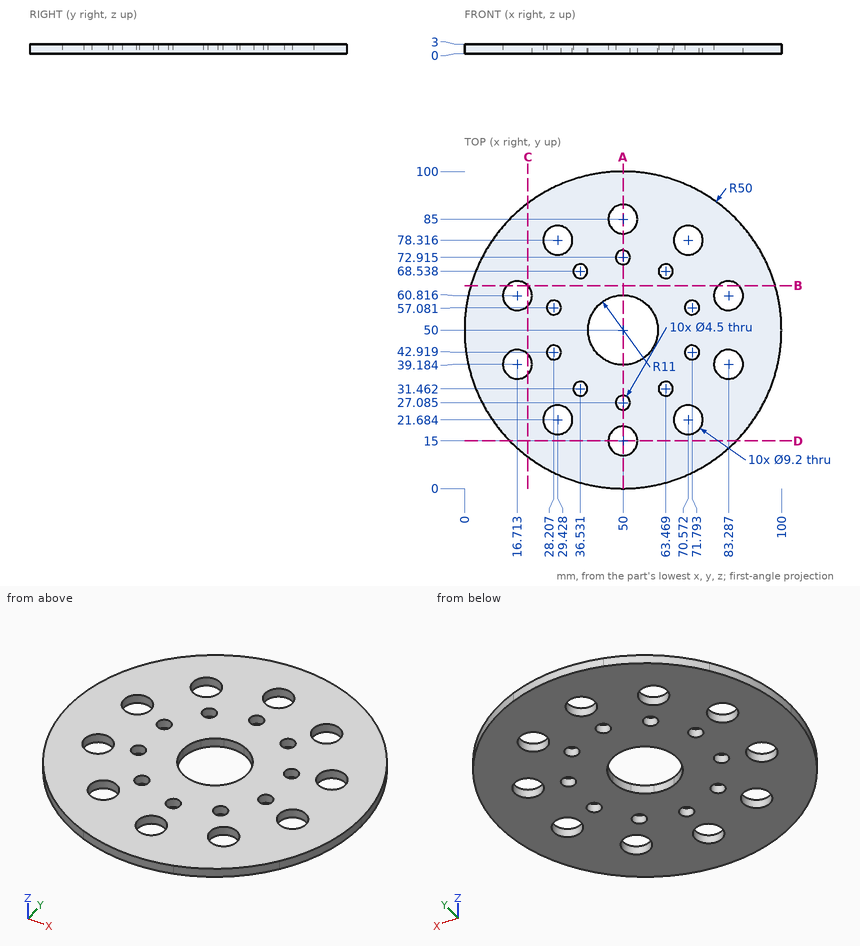
Print and shaded views of the part. All mm, measured from the part's lowest x, y and z. Coordinates: 2 decimals unless noted, no trailing zeros. Loops run counter-clockwise (first coordinate to the right, second up) from the corner with the lowest first, then second, coordinate; pieces in that order, holes last. Notation, with made-up numbers: (59.25, 68) - (88.25, 68) arc R22 cw to (88.25, 102) - close; hole circle Ø2 at (17.25, -38.5). An arc over 180 degrees is marked (long way). Use one line per item in the form item = value. Start each with the question number.
1) Drill centre lines: L1, parallel to Y at x = 50, z = 2.35 (1 decimal); L2, parallel to X at y = 75.5, z = 1.25 (1 decimal); L3, parallel to Y at x = 87, z = 0.65. Where is each one in solid material? Low to high. Write a range as from..to.
2) Band-saw the part on C-C (x = 20). Give the cut face in (y, z).
3) Band-saw the part on B-B (y = 64). Give the cut face in (x, z).
4) Flat gauge pin, fed straight in: pin 1 (1 mm diameter, centred on x = 39, z = 0.5, fed in from +Y) (1 decimal). Where does the tip first touch, or does it go through?
5) Band-saw the part on D-D (y = 15). Give the cut face in (x, z).
6) Band-saw the part on A-A (x = 50). Give the cut face in (y, z) (1 decimal), and give its area (3 significant figures).
Check values:
q1.L1 = 0..10.4, 19.6..24.8, 29.3..39, 61..70.7, 75.2..80.4, 89.6..100
q1.L2 = 7..25.8, 33.1..66.9, 74.2..93
q1.L3 = 16.37..36.47, 41.9..58.1, 63.53..83.63
q2.outline = (10, 0) - (35.97, 0) - (35.97, 3) - (10, 3) - close; (42.4, 0) - (57.6, 0) - (57.6, 3) - (42.4, 3) - close; (64.03, 0) - (90, 0) - (90, 3) - (64.03, 3) - close
q3.outline = (2, 0) - (13.39, 0) - (13.39, 3) - (2, 3) - close; (20.03, 0) - (79.97, 0) - (79.97, 3) - (20.03, 3) - close; (86.61, 0) - (98, 0) - (98, 3) - (86.61, 3) - close
q4.pin_1 = 98.9
q5.outline = (14.29, 0) - (45.4, 0) - (45.4, 3) - (14.29, 3) - close; (54.6, 0) - (85.71, 0) - (85.71, 3) - (54.6, 3) - close
q6.outline = (0, 0) - (10.4, 0) - (10.4, 3) - (0, 3) - close; (19.6, 0) - (24.8, 0) - (24.8, 3) - (19.6, 3) - close; (29.3, 0) - (39, 0) - (39, 3) - (29.3, 3) - close; (61, 0) - (70.7, 0) - (70.7, 3) - (61, 3) - close; (75.2, 0) - (80.4, 0) - (80.4, 3) - (75.2, 3) - close; (89.6, 0) - (100, 0) - (100, 3) - (89.6, 3) - close
q6.area = 152 mm2
